```python
from build123d import *

# Parameters (mm, degrees)
BOSS_EXTRUDE1_START      = 115
SKETCH2_R                = 22.5
SKETCH2_R_2              = 2.15
BOSS_EXTRUDE1_DEPTH      = 6.35
SKETCH2_4_R              = 44.45
SKETCH2_4_R_2            = 35
BOSS_EXTRUDE2_DEPTH      = 6.35
SKETCH3_W                = 1.65
SKETCH3_H                = 6.35
CIRPATTERN1_COUNT        = 12
BOSS_EXTRUDE3_DEPTH      = 6.35
BOSS_EXTRUDE4_START      = 115
BOSS_EXTRUDE4_DEPTH      = 6.35
BOSS_EXTRUDE5_DEPTH      = 22.5
BOSS_EXTRUDE5_DEPTH_BACK = 22.5


with BuildPart() as part:
    # Sketch2 → Boss-Extrude1 (new body)
    with BuildSketch(Plane.XY.offset(BOSS_EXTRUDE1_START)):
        Circle(SKETCH2_R)
        with Locations((0, 18.5)):
            Circle(SKETCH2_R_2, mode=Mode.SUBTRACT)
        with Locations((16.02146997, 9.25)):
            Circle(SKETCH2_R_2, mode=Mode.SUBTRACT)
        with Locations((16.02146997, -9.25)):
            Circle(SKETCH2_R_2, mode=Mode.SUBTRACT)
        with Locations((-16.02146997, 9.25)):
            Circle(SKETCH2_R_2, mode=Mode.SUBTRACT)
        with Locations((-16.02146997, -9.25)):
            Circle(SKETCH2_R_2, mode=Mode.SUBTRACT)
        with Locations((0, -18.5)):
            Circle(SKETCH2_R_2, mode=Mode.SUBTRACT)
    extrude(amount=BOSS_EXTRUDE1_DEPTH)

    # Sketch4<4> → Boss-Extrude4 (add)
    with BuildSketch(Plane.XY.offset(BOSS_EXTRUDE4_START)):
        with BuildLine():
            Line((-22.5, 54.45), (-22.5, 38.334742728))
            ThreePointArc((-22.5, 38.334742728), (0, 44.45), (22.5, 38.334742728))
            Line((22.5, 38.334742728), (22.5, 54.45))
            Line((22.5, 54.45), (-22.5, 54.45))
        make_face()
        with BuildLine():
            Line((-22.5, 38.334742728), (-22.5, 0))
            ThreePointArc((-22.5, 0), (0, 22.5), (22.5, 0))
            Line((22.5, 0), (22.5, 38.334742728))
            ThreePointArc((22.5, 38.334742728), (0, 44.45), (-22.5, 38.334742728))
        make_face()
    extrude(amount=BOSS_EXTRUDE4_DEPTH)



with BuildPart() as body_2:
    # Sketch2<4> → Boss-Extrude2 (new body)
    with BuildSketch(Plane.XY):
        Circle(SKETCH2_4_R)
        Circle(SKETCH2_4_R_2, mode=Mode.SUBTRACT)
    extrude(amount=BOSS_EXTRUDE2_DEPTH)

    # Sketch3 → M4x0.7 Tapped Hole1 (revolve, cut)
    with BuildSketch(Plane(origin=(0, 38, 6.35), x_dir=(0, -1, 0), z_dir=(1, 0, 0))):
        with Locations((0.825, 3.175)):
            Rectangle(SKETCH3_W, SKETCH3_H)
    m4x0_7_tapped_hole1 = revolve(axis=Axis((0, 38, 12.7), (0, 0, -1)), mode=Mode.SUBTRACT)

    # CirPattern1: M4x0.7 Tapped Hole1 ×12 about axis
    cirpattern1_axis = Axis((0, 0, 0), (0, 0, 1))
    for i in range(1, CIRPATTERN1_COUNT):
        add(m4x0_7_tapped_hole1.rotate(cirpattern1_axis, i * 360 / CIRPATTERN1_COUNT), mode=Mode.SUBTRACT)

    # Sketch4 → Boss-Extrude3 (add)
    with BuildSketch(Plane.XY):
        with BuildLine():
            Line((-39.770338523, 19.852523108), (-22.5, 54.45))
            Line((-22.5, 54.45), (22.5, 54.45))
            Line((22.5, 54.45), (39.770338523, 19.852523108))
            ThreePointArc((39.770338523, 19.852523108), (0, 44.45), (-39.770338523, 19.852523108))
        make_face()
    extrude(amount=BOSS_EXTRUDE3_DEPTH)


with BuildPart() as part_1:
    add(part.part)

    add(body_2.part)  # Boss-Extrude5 merges body 2
    # Sketch5 → Boss-Extrude5 (add, two sides: drawn at the far end of the back side and taken through both)
    with BuildSketch(Plane(origin=(0, 0, 0), x_dir=(0, 0, -1), z_dir=(1, 0, 0)).offset(-BOSS_EXTRUDE5_DEPTH_BACK)):
        with BuildLine():
            Line((0, 54.45), (0, 60.975))
            ThreePointArc((0, 60.975), (-0.878679656, 63.096320344), (-3, 63.975))
            Line((-3, 63.975), (-118.35, 63.975))
            ThreePointArc((-118.35, 63.975), (-120.471320344, 63.096320344), (-121.35, 60.975))
            Line((-121.35, 60.975), (-121.35, 54.45))
            Line((-121.35, 54.45), (-115, 54.45))
            Line((-115, 54.45), (-115, 54.625))
            ThreePointArc((-115, 54.625), (-114.121320344, 56.746320344), (-112, 57.625))
            Line((-112, 57.625), (-9.35, 57.625))
            ThreePointArc((-9.35, 57.625), (-7.228679656, 56.746320344), (-6.35, 54.625))
            Line((-6.35, 54.625), (-6.35, 54.45))
            Line((-6.35, 54.45), (0, 54.45))
        make_face()
    extrude(amount=BOSS_EXTRUDE5_DEPTH + BOSS_EXTRUDE5_DEPTH_BACK)


solid = part_1.part
```
Part model, mm, in its own coordinate system. A direction names the side the tool comes from. Round coordinates to 2 decimals unless told otherwise and drop trailing zeros. Write each loop counter-clockwise with the first axis right and the second up, starting at its lowest first coordinate (ties: lowest second). Pieces come first, ordered by that corner, then holes. Notation, with made-up numbers: M 64.5,12.5 L 116.5,12.5 A20 ccw 116.5,16.5 Z; hole C 26.5,-23 d8. An arc over 180 degrees is marked long. Answer as CSV lines item,"result". Start each with the question number.
1) Band-saw the part on C-C (y = 23). List the corners of the cut face in (x, z).
2) Drill centre lines: L1, parallel to Z at x = -21, y = 37; L2, parallel to Y at x = -19, z = 47.5 (3 decimals); L3, parallel to Z at x = 17, y = 25. Where is each one in solid material? Low to high.
3) Drop flat-ended pins along their axis: pin 1 (1 mm diameter, centred on x = 8, y = 32.5, fed in from -Z); pin 2 (4 mm diameter, centred on x = 33.5, y = 19.5, fed in from +Z); pin 3 (12 mm diameter, centred on x = -21.5, z = 42, fed in from -Y) (3 decimals). Give the stop position or say it passes through.
4) Which spindle directions (+Z, -Z, +X, -X, +Y, -Y) get a long thin tool onto all of the face, cutting with end or side? Do faces 5 (the face through (0, 16, 115)), 6 (the face through (31.273, -18.785, 3.131)), 7 (the face through (18.785, 31.273, 3.131)). Say none if no direction does.
5) Mould opens along Z. For faces 1 (the face through (-17.78, 34.02, 3.13)), 2 (the face through (10, 35, 6.35)), 3 (the face through (-0.32, 63.12, 120.45)), 4 (the face through (-4, 35, 0)) say: +Z half, -Z half, draft (parallel to the pull), parting line (faces both ways), or undercut.
6) Band-saw the part on A-A (x = 27.5). List the corners of the cut face in (y, z).
7) Band-saw the part on B-B (y = -24.5). List the corners of the cut face in (x, z) (3 decimals).
8) Band-saw the part on D-D (z = 82). List the corners of the cut face in (x, y) (3 decimals), then the cut area to 3 significant figures.
Worked out:
1,outline,"M -38.2,0 L -26.38,0 L -26.38,6.35 L -38.2,6.35 Z; M -22.5,115 L 22.5,115 L 22.5,121.35 L -22.5,121.35 Z; M 26.38,0 L 38.2,0 L 38.2,6.35 L 26.38,6.35 Z"
2,L1,"0 to 6.35, 115 to 121.35"
2,L2,"57.625 to 63.975"
2,L3,"115 to 121.35"
3,pin 1,"z = 115"
3,pin 2,"z = 6.35"
3,pin 3,"y = 57.625"
4,face 5,"+X, -X, -Y"
4,face 6,"+Z, -Z"
4,face 7,"-Z"
5,face 1,"draft"
5,face 2,"undercut"
5,face 3,"+Z half"
5,face 4,"-Z half"
6,outline,"M -34.92,0 L -21.65,0 L -21.65,6.35 L -34.92,6.35 Z; M 21.65,0 L 44.43,0 L 44.43,6.35 L 21.65,6.35 Z"
7,outline,"M -37.088,0 L -24.995,0 L -24.995,6.35 L -37.088,6.35 Z; M 24.995,0 L 37.088,0 L 37.088,6.35 L 24.995,6.35 Z"
8,outline,"M -22.5,57.625 L 22.5,57.625 L 22.5,63.975 L -22.5,63.975 Z"
8,area,"286 mm²"
